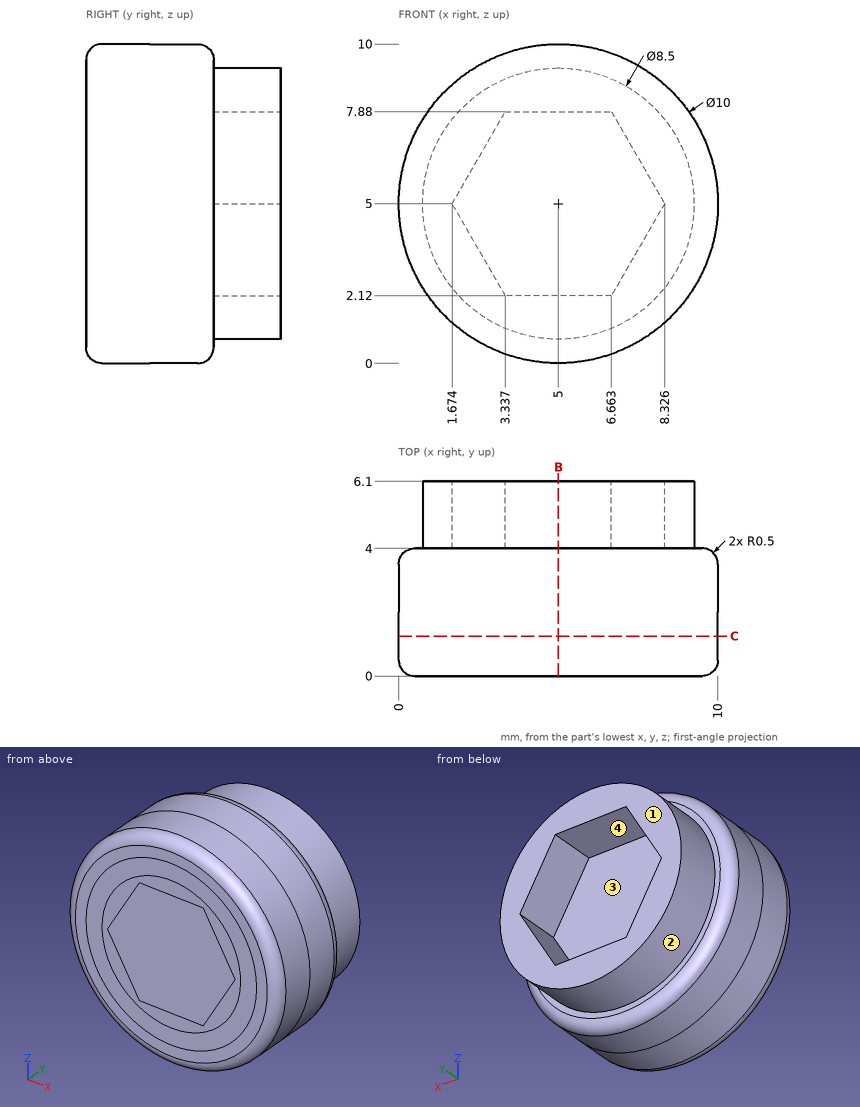
Can you work these out from the drawing? Everything is in mm from the part's minimum corner. Round coordinates to 2 decimals unless told otherwise and drop trailing zeros. Order: outer loops, then holes, each group sorted by start corner. A loop starts at its lowest first (then second) coordinate and runs counter-clockwise, first axis right, second up. Notation, with made-up numbers: (52, 75.5) -> (86, 75.5) arc R8 ccw to (86, 89.5) -> close; hole circle Ø6 at (57, 61). An arc over 180 degrees is marked (long way). Return JSON: item names as keys, results as strings. Group by question number.
1. I need wall thicknesses on line 1 (Y direction, x = 3, z = 7); line 2 (Z direction, x = 1, y = 0.5); line 3 (Z direction, x = 6, y = 5.25). Which ranges of each line are inside material? Lowest first, please. Write a range as [from, to].
2. Will these pins go through, and if not, where does the flat tip stop? pin 1 (0.6 mm diameter, centred on x = 5, y = 4.5, fed in from -Z); pin 2 (0.6 mm diameter, centred on x = 5, y = 5, fed in from +Z); pin 3 (2 mm diameter, centred on x = 8.5, y = 1.5, fed in from +Z).
3. We'd pull the mould along X, two halves only. Please class the marked faces 1, 2, 3 and 4: released by +X, released by -X, zero draft, split by the parting line, or undercut.
4. If we section it at B-B, the plane x = 5: Write out the boundary of the cut face in (y, z).
5. If we section it at C-C, the plane y = 1.25: Write out the boundary of the cut face in (x, z).
Output values:
{
 "1": {"line 1": "[0, 4]", "line 2": "[2, 8]", "line 3": "[0.87, 2.12], [7.88, 9.13]"},
 "2": {"pin 1": "z = 0.75", "pin 2": "z = 9.25", "pin 3": "z = 9.33"},
 "3": {"face 1": "zero draft", "face 2": "split by the parting line", "face 3": "undercut", "face 4": "undercut"},
 "4": {"outline": "(0, 0.5) arc R0.5 ccw to (0.5, 0) -> (3.5, 0) arc R0.5 ccw to (4, 0.5) -> (4, 0.75) -> (6.1, 0.75) -> (6.1, 2.12) -> (4, 2.12) -> (4, 7.88) -> (6.1, 7.88) -> (6.1, 9.25) -> (4, 9.25) -> (4, 9.5) arc R0.5 ccw to (3.5, 10) -> (0.5, 10) arc R0.5 ccw to (0, 9.5) -> close"},
 "5": {"outline": "circle Ø10 at (5, 5)"}
}
